```python
from build123d import *

# Parameters (mm, degrees)
SKETCH1_W                   = 2.54
SKETCH1_H                   = 2.5
SKETCH1_W_2                 = 1
SKETCH1_H_2                 = 1
BOSS_EXTRUDE1_DEPTH         = 8.35
CHAMFER1_SIZE               = 0.2
CHAMFER1_SIZE2              = 0.115470054
LPATTERN2_COUNT             = 6
LPATTERN2_PITCH             = 2.54
CHAMFER1_OF_LPATTERN2_SIZE2 = 0.115470054
CHAMFER1_OF_LPATTERN2_SIZE  = 0.2
SKETCH4_W                   = 1.2
SKETCH4_H                   = 1.2
CUT_EXTRUDE1_DEPTH          = 18.422473992
SKETCH3_W                   = 0.7
SKETCH3_H                   = 0.4
SKETCH3_W_2                 = 0.6
BOSS_EXTRUDE2_DEPTH         = 0.2
SKETCH3_3_W                 = 0.6
SKETCH3_3_H                 = 0.4
BOSS_EXTRUDE3_DEPTH         = 4.45
FILLET1_R                   = 0.1
FILLET2_R                   = 0.25
LPATTERN3_START             = -0.2
LPATTERN3_DEPTH             = 0.4
LPATTERN3_START_2           = -1
LPATTERN3_2_DEPTH           = 12


with BuildPart() as part:
    # Sketch1 → Boss-Extrude1 (new body)
    with BuildSketch(Plane.XY):
        with Locations((0.02, 0)):
            Rectangle(SKETCH1_W, SKETCH1_H)
        with Locations((0.02, 0)):
            Rectangle(SKETCH1_W_2, SKETCH1_H_2, mode=Mode.SUBTRACT)
    boss_extrude1 = extrude(amount=BOSS_EXTRUDE1_DEPTH)

    # Chamfer1
    chamfer1_edges = [part.edges().sort_by_distance(p)[0] for p in [
        (-0.48, 0, 8.35),
        (0.02, -0.5, 8.35),
        (0.52, 0, 8.35),
        (0.02, 0.5, 8.35),
    ]]
    chamfer1_side = [part.faces().sort_by_distance(p)[0] for p in [
        (0.02, -1.214360696, 8.35),
    ]]
    chamfer(chamfer1_edges, length=CHAMFER1_SIZE, length2=CHAMFER1_SIZE2, reference=chamfer1_side[0])

    # LPattern2: Boss-Extrude1 ×6
    with Locations(*[(i * LPATTERN2_PITCH, 0, 0) for i in range(1, LPATTERN2_COUNT)]):
        add(boss_extrude1)

    # Chamfer1 of LPattern2
    chamfer1_of_lpattern2_edges = [part.edges().sort_by_distance(p)[0] for p in [
        (2.06, 0, 8.35),
        (2.56, -0.5, 8.35),
        (3.06, 0, 8.35),
        (2.56, 0.5, 8.35),
        (4.6, 0, 8.35),
        (5.1, -0.5, 8.35),
        (5.6, 0, 8.35),
        (5.1, 0.5, 8.35),
        (7.14, 0, 8.35),
        (7.64, -0.5, 8.35),
        (8.14, 0, 8.35),
        (7.64, 0.5, 8.35),
        (9.68, 0, 8.35),
        (10.18, -0.5, 8.35),
        (10.68, 0, 8.35),
        (10.18, 0.5, 8.35),
        (12.22, 0, 8.35),
        (12.72, -0.5, 8.35),
        (13.22, 0, 8.35),
        (12.72, 0.5, 8.35),
    ]]
    chamfer(chamfer1_of_lpattern2_edges, length=CHAMFER1_OF_LPATTERN2_SIZE, length2=CHAMFER1_OF_LPATTERN2_SIZE2)

    # Sketch4 → Cut-Extrude1 (cut, through all)
    with BuildSketch(Plane.ZY.offset(1.25)):
        with Locations((0.6, 0)):
            Rectangle(SKETCH4_W, SKETCH4_H)
    extrude(amount=-CUT_EXTRUDE1_DEPTH, mode=Mode.SUBTRACT)

    # Sketch3 → Boss-Extrude2 (add)
    with BuildSketch(Plane(origin=(0, 0, 1.2), x_dir=(-1, 0, 0), z_dir=(0, 0, -1))):
        with Locations((-13.37, 0)):
            Rectangle(SKETCH3_W, SKETCH3_H)
        with Locations((-12.07, 0)):
            Rectangle(SKETCH3_W, SKETCH3_H)
        with Locations((-12.72, 0)):
            Rectangle(SKETCH3_W_2, SKETCH3_H)
    extrude(amount=BOSS_EXTRUDE2_DEPTH)

    # Sketch3<3> → Boss-Extrude3 (add)
    with BuildSketch(Plane(origin=(0, 0, 1.2), x_dir=(-1, 0, 0), z_dir=(0, 0, -1))):
        with Locations((-12.72, 0)):
            Rectangle(SKETCH3_3_W, SKETCH3_3_H)
    extrude(amount=BOSS_EXTRUDE3_DEPTH)

    # Fillet1
    fillet1_edges = [part.edges().sort_by_distance(p)[0] for p in [
        (12.42, 0, -3.25),
        (12.72, -0.2, -3.25),
        (12.72, 0.2, -3.25),
        (13.02, 0, -3.25),
    ]]
    fillet(fillet1_edges, radius=FILLET1_R)

    # Fillet2
    # the kernel refuses this fillet: 0.25 mm, written as the material it adds along each edge
    with BuildSketch(Plane(origin=(13.02, -0.2, 1), x_dir=(0, 0, -1), z_dir=(0, 1, 0)), Plane(origin=(12.42, 0.2, 1), x_dir=(0, 0, -1), z_dir=(0, -1, 0))) as fillet2_piece_1:
        with BuildLine():
            CenterArc((FILLET2_R, -FILLET2_R), FILLET2_R, 90, 90)
            Line((0, -FILLET2_R), (0, 0))
            Line((0, 0), (FILLET2_R, 0))
        make_face()
    extrude(amount=0.4)
    # the kernel refuses this fillet: 0.25 mm, written as the material it takes off along each edge
    with BuildSketch(Plane(origin=(11.72, -0.812372436, 1), x_dir=(1, 0, 0), z_dir=(0, 1, 0))) as fillet2_2_piece_1_section:
        with BuildLine():
            CenterArc((0.244948974, -0.25), FILLET2_R, 90, 78.463040967)
            Line((0, -0.2), (0, 0))
            Line((0, 0), (0.244948974, 0))
        make_face()
    fillet2_2_piece_1 = extrude(amount=1.624744871, mode=Mode.PRIVATE)
    fillet2_2_piece_1 = split(fillet2_2_piece_1, bisect_by=Plane(origin=(11.72, -0.6, 1), z_dir=(0, 1, 0)), keep=Keep.TOP, mode=Mode.PRIVATE)
    fillet2_2_piece_1 = split(fillet2_2_piece_1, bisect_by=Plane(origin=(11.72, 0.6, 1), z_dir=(0, -1, 0)), keep=Keep.TOP, mode=Mode.PRIVATE)
    add(fillet2_2_piece_1, mode=Mode.SUBTRACT)
    with BuildSketch(Plane(origin=(13.72, 0.812372436, 1), x_dir=(-1, 0, 0), z_dir=(0, -1, 0))) as fillet2_2_piece_2_section:
        with BuildLine():
            CenterArc((0.244948974, -0.25), FILLET2_R, 90, 78.463040967)
            Line((0, -0.2), (0, 0))
            Line((0, 0), (0.244948974, 0))
        make_face()
    fillet2_2_piece_2 = extrude(amount=1.624744871, mode=Mode.PRIVATE)
    fillet2_2_piece_2 = split(fillet2_2_piece_2, bisect_by=Plane(origin=(13.72, -0.6, 1), z_dir=(0, 1, 0)), keep=Keep.TOP, mode=Mode.PRIVATE)
    fillet2_2_piece_2 = split(fillet2_2_piece_2, bisect_by=Plane(origin=(13.72, 0.6, 1), z_dir=(0, -1, 0)), keep=Keep.TOP, mode=Mode.PRIVATE)
    add(fillet2_2_piece_2, mode=Mode.SUBTRACT)

    # LPattern3: read off the stored shape, not the designer's step
    # LPattern3 outline → LPattern3 (add)
    with BuildSketch(Plane(origin=(0, 0, 0), x_dir=(1, 0, 0), z_dir=(0, 1, 0)).offset(LPATTERN3_START)):
        with BuildLine():
            ThreePointArc((9.424948974, -1), (9.266835091, -1.056350833), (9.18, -1.2))
            Line((9.18, -1.2), (11.18, -1.2))
            ThreePointArc((11.18, -1.2), (11.093164909, -1.056350833), (10.935051026, -1))
            Line((10.935051026, -1), (10.73, -1))
            ThreePointArc((10.73, -1), (10.553223305, -0.926776695), (10.48, -0.75))
            Line((10.48, -0.75), (10.48, 3.15))
            ThreePointArc((10.48, 3.15), (10.450710678, 3.220710678), (10.38, 3.25))
            Line((10.38, 3.25), (9.98, 3.25))
            ThreePointArc((9.98, 3.25), (9.909289322, 3.220710678), (9.88, 3.15))
            Line((9.88, 3.15), (9.88, -0.75))
            ThreePointArc((9.88, -0.75), (9.806776695, -0.926776695), (9.63, -1))
            Line((9.63, -1), (9.424948974, -1))
        make_face()
        with BuildLine():
            ThreePointArc((6.884948974, -1), (6.726835091, -1.056350833), (6.64, -1.2))
            Line((6.64, -1.2), (8.64, -1.2))
            ThreePointArc((8.64, -1.2), (8.553164909, -1.056350833), (8.395051026, -1))
            Line((8.395051026, -1), (8.19, -1))
            ThreePointArc((8.19, -1), (8.013223305, -0.926776695), (7.94, -0.75))
            Line((7.94, -0.75), (7.94, 3.15))
            ThreePointArc((7.94, 3.15), (7.910710678, 3.220710678), (7.84, 3.25))
            Line((7.84, 3.25), (7.44, 3.25))
            ThreePointArc((7.44, 3.25), (7.369289322, 3.220710678), (7.34, 3.15))
            Line((7.34, 3.15), (7.34, -0.75))
            ThreePointArc((7.34, -0.75), (7.266776695, -0.926776695), (7.09, -1))
            Line((7.09, -1), (6.884948974, -1))
        make_face()
        with BuildLine():
            ThreePointArc((4.344948974, -1), (4.186835091, -1.056350833), (4.1, -1.2))
            Line((4.1, -1.2), (6.1, -1.2))
            ThreePointArc((6.1, -1.2), (6.013164909, -1.056350833), (5.855051026, -1))
            Line((5.855051026, -1), (5.65, -1))
            ThreePointArc((5.65, -1), (5.473223305, -0.926776695), (5.4, -0.75))
            Line((5.4, -0.75), (5.4, 3.15))
            ThreePointArc((5.4, 3.15), (5.370710678, 3.220710678), (5.3, 3.25))
            Line((5.3, 3.25), (4.9, 3.25))
            ThreePointArc((4.9, 3.25), (4.829289322, 3.220710678), (4.8, 3.15))
            Line((4.8, 3.15), (4.8, -0.75))
            ThreePointArc((4.8, -0.75), (4.726776695, -0.926776695), (4.55, -1))
            Line((4.55, -1), (4.344948974, -1))
        make_face()
        with BuildLine():
            ThreePointArc((1.804948974, -1), (1.646835091, -1.056350833), (1.56, -1.2))
            Line((1.56, -1.2), (3.56, -1.2))
            ThreePointArc((3.56, -1.2), (3.473164909, -1.056350833), (3.315051026, -1))
            Line((3.315051026, -1), (3.11, -1))
            ThreePointArc((3.11, -1), (2.933223305, -0.926776695), (2.86, -0.75))
            Line((2.86, -0.75), (2.86, 3.15))
            ThreePointArc((2.86, 3.15), (2.830710678, 3.220710678), (2.76, 3.25))
            Line((2.76, 3.25), (2.36, 3.25))
            ThreePointArc((2.36, 3.25), (2.289289322, 3.220710678), (2.26, 3.15))
            Line((2.26, 3.15), (2.26, -0.75))
            ThreePointArc((2.26, -0.75), (2.186776695, -0.926776695), (2.01, -1))
            Line((2.01, -1), (1.804948974, -1))
        make_face()
        with BuildLine():
            Line((0.775051026, -1), (0.57, -1))
            ThreePointArc((0.57, -1), (0.393223305, -0.926776695), (0.32, -0.75))
            Line((0.32, -0.75), (0.32, 3.15))
            ThreePointArc((0.32, 3.15), (0.290710678, 3.220710678), (0.22, 3.25))
            Line((0.22, 3.25), (-0.18, 3.25))
            ThreePointArc((-0.18, 3.25), (-0.250710678, 3.220710678), (-0.28, 3.15))
            Line((-0.28, 3.15), (-0.28, -0.75))
            ThreePointArc((-0.28, -0.75), (-0.353223305, -0.926776695), (-0.53, -1))
            Line((-0.53, -1), (-0.735051026, -1))
            ThreePointArc((-0.735051026, -1), (-0.893164909, -1.056350833), (-0.98, -1.2))
            Line((-0.98, -1.2), (1.02, -1.2))
            ThreePointArc((1.02, -1.2), (0.933164909, -1.056350833), (0.775051026, -1))
        make_face()
    extrude(amount=LPATTERN3_DEPTH)

    # LPattern3 2 outline → LPattern3 2 (cut)
    with BuildSketch(Plane.YZ.offset(LPATTERN3_START_2)):
        with BuildLine():
            Line((0.2, -3.25), (0.2, -3.15))
            ThreePointArc((0.2, -3.15), (0.170710678, -3.220710678), (0.1, -3.25))
            Line((0.1, -3.25), (0.2, -3.25))
        make_face()
        with BuildLine():
            Line((-0.2, -3.25), (-0.1, -3.25))
            ThreePointArc((-0.1, -3.25), (-0.170710678, -3.220710678), (-0.2, -3.15))
            Line((-0.2, -3.15), (-0.2, -3.25))
        make_face()
    extrude(amount=LPATTERN3_2_DEPTH, mode=Mode.SUBTRACT)


solid = part.part
```
CAD build for the part. Positions are in the model's coordinates, mm. A direction names the side the tool comes from. Round coordinates to 2 decimals unless told otherwise and drop trailing zeros. Write each loop counter-clockwise with the first axis right and the second up, starting at its lowest first coordinate (ties: lowest second). Pieces come first, ordered by that corner, then holes. Notation, with made-up numbers: (83, -17.5) - (141, -17.5) arc R30 ccw to (141, 13.5) - close; hole circle Ø7 at (-8.75, -35.75). An arc over 180 degrees is marked (long way). Return JSON: item names as keys, results as strings. Group by question number.
Item 1: Band-saw the part on B-B on z = 6.5. List the corners of the cut face in (x, y).
Item 2: Probe probe 1 along Y at (x, z) = (-0.25, 1); probe 2 along Y at (x, z) = (2.5, 8); probe 3 along Z at (x, y) = (4, -0.4). List the from-to ranges inside material, lowest first.
Item 3: 3-axis set-ups, long thin cutter, end or side, ignore diameter. For faces 3 (the face through (0, -0.5, 5)), 4 (the face through (4.6, 0, 5)), 5 (the face through (6, -0.6, 1)): which of +Z, -Z, +X, -X, +Y, -Y reach the whole face in a straight line?
Item 4: Band-saw the part on C-C on z = 0.5. State how many separate pieces and enclosed holes the cut face has, plus the area to 3 significant figures.
Item 5: Band-saw the part on D-D on y = -0.9. List the corners of the cut face in (x, z).
Item 6: Band-saw the part on A-A on z = -2. List the corners of the cut face in (x, y), plus the area to 3 significant figures.
Item 7: Mould opens along X. For faces 1 (the face through (13, -0.5, 5)), 2 (the face through (6, 1.25, 4)) say: +X half, -X half, draft (parallel to the pull), parting line (faces both ways), or undercut.
Resolved:
{
 "1": {"outline": "(-1.25, -1.25) - (13.99, -1.25) - (13.99, 1.25) - (-1.25, 1.25) - close; hole (-0.48, -0.5) - (0.52, -0.5) - (0.52, 0.5) - (-0.48, 0.5) - close; hole (2.06, -0.5) - (3.06, -0.5) - (3.06, 0.5) - (2.06, 0.5) - close; hole (4.6, -0.5) - (5.6, -0.5) - (5.6, 0.5) - (4.6, 0.5) - close; hole (7.14, -0.5) - (8.14, -0.5) - (8.14, 0.5) - (7.14, 0.5) - close; hole (9.68, -0.5) - (10.68, -0.5) - (10.68, 0.5) - (9.68, 0.5) - close; hole (12.22, -0.5) - (13.22, -0.5) - (13.22, 0.5) - (12.22, 0.5) - close"},
 "2": {"probe 1": "y = -1.25 to -0.6, -0.2 to 0.2, 0.6 to 1.25", "probe 2": "y = -1.25 to -0.5, 0.5 to 1.25", "probe 3": "z = 1.2 to 8.35"},
 "3": {"face 3": "+Z, -Z", "face 4": "+Z", "face 5": "-Z, +X, -X"},
 "4": {"separate pieces": "8", "enclosed holes": "0", "area": "21.3 mm²"},
 "5": {"outline": "(-1.25, 0) - (13.99, 0) - (13.99, 8.35) - (-1.25, 8.35) - close"},
 "6": {"outline": "(-0.28, -0.2) - (0.32, -0.2) - (0.32, 0.2) - (-0.28, 0.2) - close; (2.26, -0.2) - (2.86, -0.2) - (2.86, 0.2) - (2.26, 0.2) - close; (4.8, -0.2) - (5.4, -0.2) - (5.4, 0.2) - (4.8, 0.2) - close; (7.34, -0.2) - (7.94, -0.2) - (7.94, 0.2) - (7.34, 0.2) - close; (9.88, -0.2) - (10.48, -0.2) - (10.48, 0.2) - (9.88, 0.2) - close; (12.42, -0.2) - (13.02, -0.2) - (13.02, 0.2) - (12.42, 0.2) - close", "area": "1.44 mm²"},
 "7": {"face 1": "undercut", "face 2": "draft"}
}
